```python
from build123d import *

# Parameters (mm, degrees)
SKETCH1_W           = 3.175
SKETCH1_H           = 3.175
BOSS_EXTRUDE1_DEPTH = 6.35


with BuildPart() as part:
    # Sketch1 → Boss-Extrude1 (new body)
    with BuildSketch(Plane.XY):
        with BuildLine():
            ThreePointArc((95.894192869, 3.526467972), (46.7995, 18.096007393), (-2.295192869, 3.526467972))
            ThreePointArc((-2.295192869, 3.526467972), (-3.526467972, -2.295192869), (2.295192869, -3.526467972))
            ThreePointArc((2.295192869, -3.526467972), (46.7995, 9.68081003), (91.303807131, -3.526467972))
            ThreePointArc((91.303807131, -3.526467972), (97.125467972, -2.295192869), (95.894192869, 3.526467972))
        make_face()
        with Locations((93.599, 0)):
            Rectangle(SKETCH1_W, SKETCH1_H, mode=Mode.SUBTRACT)
        Rectangle(SKETCH1_W, SKETCH1_H, mode=Mode.SUBTRACT)
    extrude(amount=BOSS_EXTRUDE1_DEPTH)


solid = part.part
```
Can you work these out from the model? Positions are in its coordinate system, mm. A direction names the side the tool comes from. Give positions to 0.01 mm unless a question says otherwise; leave off trailing zeros. Loops run counter-clockwise (first coordinate to the right, second up) from the corner with the lowest first, then second, coordinate; pieces in that order, holes last. Notation, with made-up numbers: M 56.5,-39 L 92.5,-39 A10 cw 92.5,-22 Z; hole C 73.5,-21 d6. An arc over 180 degrees is marked long. Use CSV: the item, a comma, the result in double quotes. Start each with the question number.
1. On a 3-axis mill with a long thin cutter (end or side, diameter ignored), from which of +Z, -Z, +X, -X, +Y, -Y can I reach the whole of each face in a straight line? I mean faces 4 (the face through (92.012, 0, 3)), 5 (the face through (46.14, 9.68, 3.13)). Say none if no direction works.
2. Imagine slicing it at A-A, the plane z = 4. Write out the boundary of the cut face in (x, y), plus the area to 3 significant figures.
3. If I drill on L1, parallel to X at y = 1, z = 4.75; L2, parallel to X at y = -0.5, z = 4; L3, parallel to Y at x = 1, z = 6.25, over which ranges is the centre line in solid material (lowest first)?
4. If we mould it in two halves opening along X, with no side actions, what happens to faces 1 (the face through (46, 12, 0)), 2 (the face through (47.526, 18.093, 3.131)), 3 (the face through (94, 1.588, 3))? For each: released by +X, released by -X, zero draft, split by the parting line, or undercut.
5. Imagine slicing it at B-B, the plane x = 0. Write out the boundary of the cut face in (y, z).
6. For P1, Ø2, axis at x = 85, z = 2, coming from the +Y side; P2, Ø1, axis at x = 93, z = 1.5, coming from the +Y side; P3, Ø1.6, axis at x = 0.5, z = 2, coming from the +Y side, each with a flat end and sliding along its axis, tell me the tip position at first contact or that it passes through.
7. Imagine slicing it at C-C, the plane y = 0. Write out the boundary of the cut face in (x, z).
8. Imagine slicing it at D-D, the plane x = 45. Write out the boundary of the cut face in (y, z), plus the area to 3 significant figures.
Response values:
1,face 4,"+Z, -Z"
1,face 5,"+Z, -Z, -Y"
2,outline,"M -2.3,3.53 A4.21 ccw 2.3,-3.53 A81.59 cw 91.3,-3.53 A4.21 ccw 95.89,3.53 A90 ccw Z; hole M -1.59,-1.59 L 1.59,-1.59 L 1.59,1.59 L -1.59,1.59 Z; hole M 92.01,-1.59 L 95.19,-1.59 L 95.19,1.59 L 92.01,1.59 Z"
2,area,"869 mm^2"
3,L1,"-4.09 to -1.59, 1.59 to 10.18, 83.42 to 92.01, 95.19 to 97.69"
3,L2,"-4.18 to -1.59, 1.59 to 7.33, 86.27 to 92.01, 95.19 to 97.78"
3,L3,"-4.09 to -1.59, 1.59 to 5.57"
4,face 1,"zero draft"
4,face 2,"split by the parting line"
4,face 3,"undercut"
5,outline,"M -4.21,0 L -1.59,0 L -1.59,6.35 L -4.21,6.35 Z; M 1.59,0 L 4.97,0 L 4.97,6.35 L 1.59,6.35 Z"
6,P1,"y = 10.05"
6,P2,"y = 5.63"
6,P3,"y = 5.75"
7,outline,"M -4.21,0 L -1.59,0 L -1.59,6.35 L -4.21,6.35 Z; M 1.59,0 L 8.25,0 L 8.25,6.35 L 1.59,6.35 Z; M 85.35,0 L 92.01,0 L 92.01,6.35 L 85.35,6.35 Z; M 95.19,0 L 97.81,0 L 97.81,6.35 L 95.19,6.35 Z"
8,outline,"M 9.66,0 L 18.08,0 L 18.08,6.35 L 9.66,6.35 Z"
8,area,"53.4 mm^2"
